The figure shows three views and two pictorial views of one solid part (mm, origin at its lowest corner). Answer the questions. Coordinates: 2 decimals unless noted, no trailing zeros. Loops run counter-clockwise (first coordinate to the right, second up) from the corner with the lowest first, then second, coordinate; pieces in that order, holes last. Notation, with made-up numbers: (-2.75, 14) - (35.25, 14) arc R24 ccw to (35.25, 48) - close; hole circle Ø8 at (12.5, 81). An arc over 180 degrees is marked (long way). Write each question's results on one line, items separated by ' | '. Start each with the question number.
Item 1: Section A-A, the plane z = 9.5 is taken. Write down the section's boundary in (x, y), plus the area to 3 significant figures.
Item 2: Section B-B, the plane x = 82.55 is taken. Write down the section's boundary in (y, z).
Item 3: For a pull along X with two mould halves and no side action, classify the marked faces 1, 2 and 3 as +X half, -X half, draft (parallel to the pull), parting line (faces both ways), or undercut.
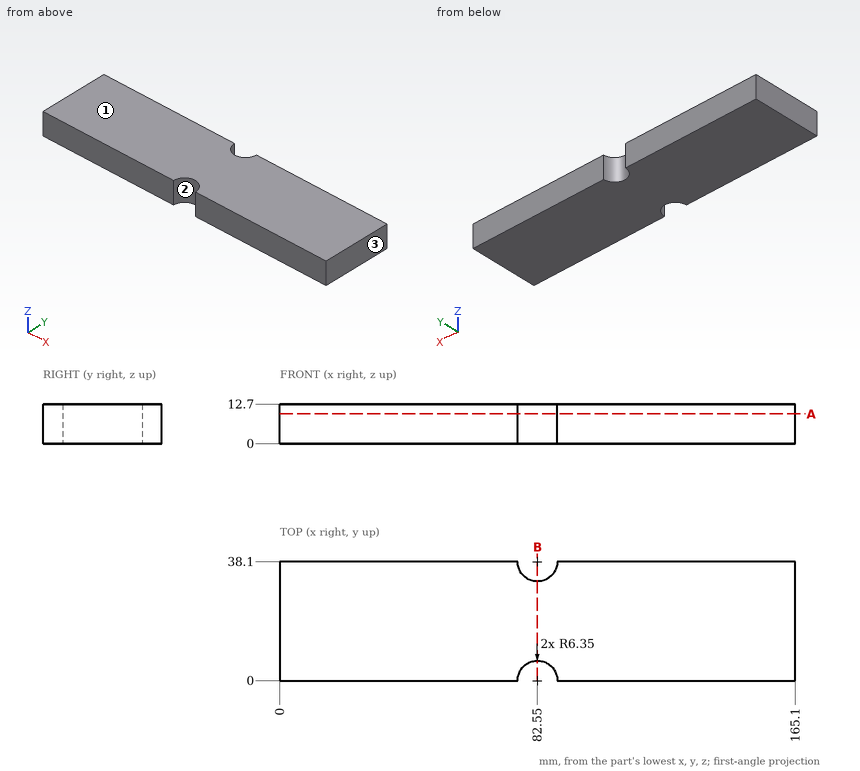
Answer key:
1) outline: (0, 0) - (76.2, 0) arc R6.35 cw to (88.9, 0) - (165.1, 0) - (165.1, 38.1) - (88.9, 38.1) arc R6.35 cw to (76.2, 38.1) - (0, 38.1) - close | area: 6,160 mm^2
2) outline: (6.35, 0) - (31.75, 0) - (31.75, 12.7) - (6.35, 12.7) - close
3) face 1: draft | face 2: undercut | face 3: +X half
